```python
from build123d import *

# Parameters (mm, degrees)
F0_W     = 40
F0_H     = 60
F0_R     = 2.25
F0_R_2   = 3.4
F0_R_3   = 4.5
F1_DEPTH = 6
F2_SIZE  = 3.75


with BuildPart() as f1:
    # F0 (on Top) → F1 (new body)
    with BuildSketch(Plane.XY):
        with Locations((20, 30)):
            Rectangle(F0_W, F0_H)
        with Locations((7, 7)):
            Circle(F0_R, mode=Mode.SUBTRACT)
        with Locations((33, 7)):
            Circle(F0_R, mode=Mode.SUBTRACT)
        with Locations((7, 53)):
            Circle(F0_R, mode=Mode.SUBTRACT)
        with Locations((20, 30)):
            Circle(F0_R_2, mode=Mode.SUBTRACT)
        with Locations((20, 50)):
            Circle(F0_R_3, mode=Mode.SUBTRACT)
        with Locations((33, 53)):
            Circle(F0_R, mode=Mode.SUBTRACT)
    extrude(amount=F1_DEPTH)

    # F2
    f2_edges = [f1.edges().sort_by_distance(p)[0] for p in [
        (4.75, 7, 6),
        (30.75, 7, 6),
        (30.75, 53, 6),
        (4.75, 53, 6),
    ]]
    chamfer(f2_edges, length=F2_SIZE)


solid = f1.part
```
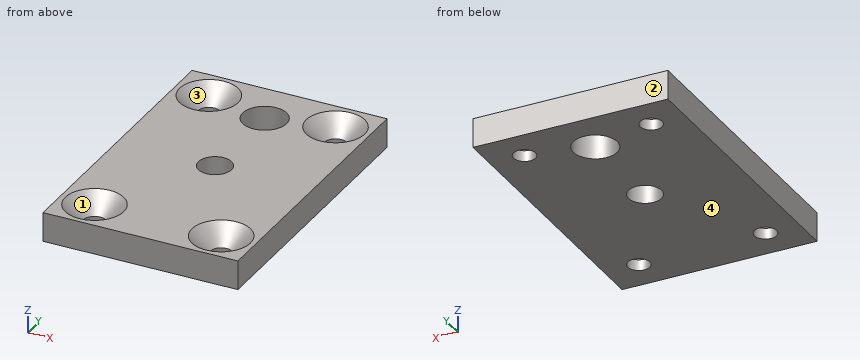
For this review, take the finished solid that the model builds, in its own axes (mm). Face numbers are marked on the shaded views. Coordinates: 2 decimals unless noted, no trailing zeros. Loops run counter-clockwise (first coordinate to the right, second up) from the corner with the lowest first, then second, coordinate; pieces in that order, holes last. Notation, with made-up numbers: (45, 71.5) -> (69, 71.5) arc R17 cw to (69, 81.5) -> close; hole circle Ø1 at (33.5, 63.5). An arc over 180 degrees is marked (long way). Return JSON: item names as keys, results as strings. Group by question number.
(1) Consider section A-A, the plane y = 30. Give the boundary of the cut face in (x, z).
(2) To check wall thickness, follow L1, parallel to Y at x = 7, z = 1.65; L2, parallel to Y at x = 20, z = 2.4; L3, parallel to X at y = 53.5, z = 1.4. State the ranges of each line that lie inside material, in increasing order.
(3) Consider section D-D, the plane z = 3.5. Give the boundary of the cut face in (x, y), plus the area to 3 significant figures.
(4) For pin 1 Ø6 at (x, y) = (20, 30) entering from -Z, flat-tipped, find the tip position at first contact; note if it passes through.
(5) Consider section C-C, the plane y = 7. Give the boundary of the cut face in (x, z).
(6) Mouldability with a two-part tool opening along Y and no side actions: class the marked faces 1, 2, 3 and 4 as pulls with the +Y half, pulls with the -Y half, needs draft (parallel to the pull), parting line crosses it, or undercut.
(7) Consider section B-B, the plane x = 33. Give the boundary of the cut face in (y, z), plus the area to 3 significant figures.
Results below:
{
 "1": {"outline": "(0, 0) -> (16.6, 0) -> (16.6, 6) -> (0, 6) -> close; (23.4, 0) -> (40, 0) -> (40, 6) -> (23.4, 6) -> close"},
 "2": {"L1": "y = 0 to 4.75, 9.25 to 50.75, 55.25 to 60", "L2": "y = 0 to 26.6, 33.4 to 45.5, 54.5 to 60", "L3": "x = 0 to 4.81, 9.19 to 17.17, 22.83 to 30.81, 35.19 to 40"},
 "3": {"outline": "(0, 0) -> (40, 0) -> (40, 60) -> (0, 60) -> close; hole circle Ø7 at (7, 7); hole circle Ø7 at (7, 53); hole circle Ø9 at (20, 50); hole circle Ø6.8 at (20, 30); hole circle Ø7 at (33, 7); hole circle Ø7 at (33, 53)", "area": "2,150 mm2"},
 "4": {"pin 1": "passes through"},
 "5": {"outline": "(0, 0) -> (4.75, 0) -> (4.75, 2.25) -> (1, 6) -> (0, 6) -> close; (9.25, 0) -> (30.75, 0) -> (30.75, 2.25) -> (27, 6) -> (13, 6) -> (9.25, 2.25) -> close; (35.25, 0) -> (40, 0) -> (40, 6) -> (39, 6) -> (35.25, 2.25) -> close"},
 "6": {"face 1": "undercut", "face 2": "pulls with the +Y half", "face 3": "undercut", "face 4": "needs draft"},
 "7": {"outline": "(0, 0) -> (4.75, 0) -> (4.75, 2.25) -> (1, 6) -> (0, 6) -> close; (9.25, 0) -> (50.75, 0) -> (50.75, 2.25) -> (47, 6) -> (13, 6) -> (9.25, 2.25) -> close; (55.25, 0) -> (60, 0) -> (60, 6) -> (59, 6) -> (55.25, 2.25) -> close", "area": "278 mm2"}
}
